The model under review builds one solid part; all positions refer to its coordinate system, in mm. A direction names the side the tool comes from. Round coordinates to 2 decimals unless told otherwise and drop trailing zeros. Write each loop counter-clockwise with the first axis right and the second up, starting at its lowest first coordinate (ties: lowest second). Pieces come first, ordered by that corner, then holes. Notation, with made-up numbers: (15, -29.75) - (31, -29.75) arc R19 cw to (31, -24.75) - close; hole circle Ø9 at (51, -12). An arc over 180 degrees is marked (long way). Return JSON: item names as keys, results as strings.
from build123d import *

# Parameters (mm, degrees)
SKETCH1_R           = 180
SKETCH1_R_2         = 150
BOSS_EXTRUDE1_DEPTH = 15
SKETCH2_R           = 165
SKETCH2_R_2         = 150
BOSS_EXTRUDE2_DEPTH = 15
CUT_EXTRUDE1_REACH  = 32
SKETCH3_W           = 245
SKETCH3_H           = 360


with BuildPart() as part:
    # Sketch1 → Boss-Extrude1 (new body)
    with BuildSketch(Plane.XY):
        Circle(SKETCH1_R)
        Circle(SKETCH1_R_2, mode=Mode.SUBTRACT)
    extrude(amount=BOSS_EXTRUDE1_DEPTH)

    # Sketch2 → Boss-Extrude2 (add)
    with BuildSketch(Plane.XY.offset(15)):
        Circle(SKETCH2_R)
        Circle(SKETCH2_R_2, mode=Mode.SUBTRACT)
    extrude(amount=BOSS_EXTRUDE2_DEPTH)

    # Sketch3 → Cut-Extrude1 (cut, up to next)
    with BuildSketch(Plane.XY, mode=Mode.PRIVATE) as cut_extrude1_sk1:
        with Locations((122.5, 0)):
            Rectangle(SKETCH3_W, SKETCH3_H)
    cut_extrude1_tool1 = extrude(cut_extrude1_sk1.sketch, amount=CUT_EXTRUDE1_REACH, mode=Mode.PRIVATE) & part.part
    add(cut_extrude1_tool1.solids().sort_by_distance((122.5, 0, 0))[0], mode=Mode.SUBTRACT)


solid = part.part
(1) Add section A-A (x = -102). Write out the cut boundary in (y, z), plus the area to 3 significant figures.
Filled in:
{"outline": "(-148.31, 0) - (-109.98, 0) - (-109.98, 30) - (-129.7, 30) - (-129.7, 15) - (-148.31, 15) - close; (109.98, 0) - (148.31, 0) - (148.31, 15) - (129.7, 15) - (129.7, 30) - (109.98, 30) - close", "area": "1,740 mm2"}
(2) Wall thickness on line 1 (Y direction, x = -88, z = 14); line 2 (Z direction, x = -171.5, y = -6); line 3 (Y direction, x = -64, z = 14.75): over which ranges is each line inside the solid? List them lowest first.
Filled in:
{"line 1": "y = -157.02 to -121.47, 121.47 to 157.02", "line 2": "z = 0 to 15", "line 3": "y = -168.24 to -135.66, 135.66 to 168.24"}
(3) Add section C-C (x = -155.5). Write out the cut boundary in (y, z), plus the area to 3 significant figures.
Filled in:
{"outline": "(-90.66, 0) - (90.66, 0) - (90.66, 15) - (55.18, 15) - (55.18, 30) - (-55.18, 30) - (-55.18, 15) - (-90.66, 15) - close", "area": "4,380 mm2"}
(4) Clearance check with flat-ended pins moving along their axes: pin 1 Ø5 at (y, z) = (-115, 23) entering from +X; pin 2 Ø4 at (y, z) = (43.5, 17) entering from +X; pin 3 Ø1.5 at (x, z) = (-79.5, 12.5) entering from -Y. State where each tip first meets the part, or that it passes through.
Filled in:
{"pin 1": "stops at x = -93.24", "pin 2": "stops at x = -142.93", "pin 3": "stops at y = -161.86"}
(5) Add section B-B (y = 0). Write out the cut boundary in (x, z), plus the area to 3 significant figures.
Filled in:
{"outline": "(-180, 0) - (-150, 0) - (-150, 30) - (-165, 30) - (-165, 15) - (-180, 15) - close", "area": "675 mm2"}
(6) For faces 1 (the flat face through (-150, 13, 30)), 2 (the cylindrical face through (-164.96, 3.63, 22.4)), list the 3-axis set-ups (+Z, -Z, +X, -X, +Y, -Y) from which the entire face can be reached by the end or side of a thin tool; tool diameter is ignored.
Filled in:
{"face 1": "+Z, +X, -X, +Y, -Y", "face 2": "+Z, -X"}
(7) Add section D-D (x = -51). Write out the cut boundary in (y, z), plus the area to 3 significant figures.
Filled in:
{"outline": "(-172.62, 0) - (-141.06, 0) - (-141.06, 30) - (-156.92, 30) - (-156.92, 15) - (-172.62, 15) - close; (141.06, 0) - (172.62, 0) - (172.62, 15) - (156.92, 15) - (156.92, 30) - (141.06, 30) - close", "area": "1,420 mm2"}
